Geometry: final body of the model. Coordinates: model frame, mm. Face numbers are marked on the shaded views. Round coordinates to 2 decimals unless told otherwise and drop trailing zeros. Loops run counter-clockwise (first coordinate to the right, second up) from the corner with the lowest first, then second, coordinate; pieces in that order, holes last. Notation, with made-up numbers: (53.25, 79) - (65.25, 79) arc R15 ccw to (65.25, 108) - close; hole circle Ø6 at (80, -5.5). An arc over 180 degrees is marked (long way). Use CSV: the item, a comma, the result in double quotes.
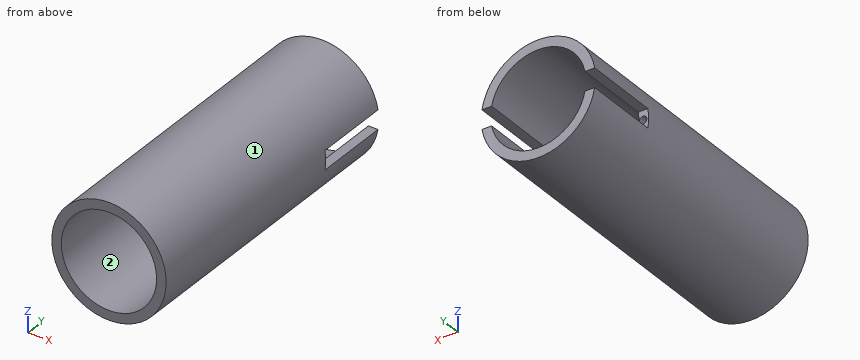
from build123d import *

# Parameters (mm, degrees)
F0_R     = 38.1
F1_DEPTH = 203.2
F2_R     = 31.75
F3_DEPTH = 228.6
F4_W     = 76.2
F4_H     = 12.7
F5_DEPTH = 50.8
F6_R     = 2.54
F7_DEPTH = 25.4


with BuildPart() as f1:
    # F0 (on Front) → F1 (new body)
    with BuildSketch(Plane.XZ):
        Circle(F0_R)
    extrude(amount=F1_DEPTH)

    # F2 (on face) → F3 (cut)
    with BuildSketch(Plane.XZ.offset(203.2)):
        Circle(F2_R)
    extrude(amount=-F3_DEPTH, mode=Mode.SUBTRACT)

    # F4 (on Front) → F5 (cut)
    with BuildSketch(Plane.XZ):
        Rectangle(F4_W, F4_H)
    extrude(amount=F5_DEPTH, mode=Mode.SUBTRACT)

    # F6 (on face) → F7 (cut)
    with BuildSketch(Plane(origin=(0, -50.8, 0), x_dir=(-1, 0, 0), z_dir=(0, 1, 0))):
        with Locations((-34.337813, 0)):
            Circle(F6_R)
        with Locations((34.337813, 0)):
            Circle(F6_R)
    extrude(amount=-F7_DEPTH, mode=Mode.SUBTRACT)


solid = f1.part
Item 1: Mould query, pull axis Z, two halves, no side actions, for the marked faces 1 and 2. Classes: released by +Z, released by -Z, zero draft, split by the parting line, or undercut.
Final values:
face 1,"split by the parting line"
face 2,"undercut"
Item 2: Pin query (flat end, axial travel): P1, Ø4, axis at x = -34, z = -1, coming from the +Y side; P2, Ø5, axis at x = 34.5, y = -36.5, coming from the -Z side; P3, Ø3, axis at x = 34, y = -25, coming from the +Z side. Return the tip coordinate at first contact, or that it passes through.
Final values:
P1,"stops at y = -50.8"
P2,"stops at z = -20.68"
P3,"stops at z = 19.88"
Item 3: Material intervals for line 1 (Z direction, x = -1, y = -38); line 2 (X direction, y = -37.5, z = 6.5); line 3 (Z direction, x = 21, y = -102), sorted ascending.
Final values:
line 1,"z = -38.09 to -31.73, 31.73 to 38.09"
line 2,"x = -37.54 to -31.08, 31.08 to 37.54"
line 3,"z = -31.79 to -23.81, 23.81 to 31.79"
Item 4: Section A-A on z = 0. Return the cut outline in (x, y).
Final values:
outline,"(-38.1, -203.2) - (-31.75, -203.2) - (-31.75, -50.8) - (-31.8, -50.8) - (-31.8, -76.2) - (-36.88, -76.2) - (-36.88, -50.8) - (-38.1, -50.8) - close; (31.75, -203.2) - (38.1, -203.2) - (38.1, -50.8) - (36.88, -50.8) - (36.88, -76.2) - (31.8, -76.2) - (31.8, -50.8) - (31.75, -50.8) - close"
Item 5: Section B-B on x = 0. Return the cut outline in (y, z), plus the area to 3 significant figures.
Final values:
outline,"(-203.2, -38.1) - (0, -38.1) - (0, -31.75) - (-203.2, -31.75) - close; (-203.2, 31.75) - (0, 31.75) - (0, 38.1) - (-203.2, 38.1) - close"
area,"2,580 mm²"
Item 6: Section D-D on y = -161.5. Return the cut outline in (x, z).
Final values:
outline,"circle Ø76.2 at (0, 0); hole circle Ø63.5 at (0, 0)"
Item 7: Section C-C on y = -23. Return the cut outline in (x, z).
Final values:
outline,"(-37.57, -6.35) arc R38.1 ccw to (37.57, -6.35) - (31.11, -6.35) arc R31.75 cw to (-31.11, -6.35) - close; (-37.57, 6.35) - (-31.11, 6.35) arc R31.75 cw to (31.11, 6.35) - (37.57, 6.35) arc R38.1 ccw to start"
